Could you check a few things on this model? Use its own coordinates, in mm. Face numbers are marked on the shaded views. A direction names the side the tool comes from. Give positions to 0.01 mm unless a question says otherwise; leave off trailing zeros. Write each loop counter-clockwise with the first axis right and the second up, starting at its lowest first coordinate (ties: lowest second). Pieces come first, ordered by that corner, then holes. Notation, with made-up numbers: M 29.25,62 L 77.25,62 A32 cw 77.25,88 Z; hole C 12.25,6.5 d11. An arc over 180 degrees is marked long. Answer as a JSON object with one key per item and string values. Group by question number.
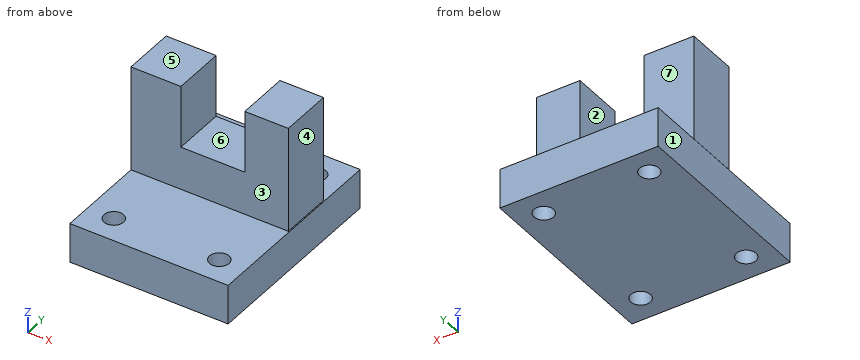
```python
from build123d import *

# Parameters (mm, degrees)
F2_W     = 0.0470026281
F2_H     = 25.4
F2_W_2   = 75.699427795
F3_DEPTH = 50.8
F1_W     = 76.2
F1_H     = 95.25
F1_R     = 4.699
F4_DEPTH = 19.05
F5_W     = 30.7534076273
F5_H     = 29.9894312948
F6_DEPTH = 31.75


with BuildPart() as f3:
    # F2 (on face) → F3 (new body)
    with BuildSketch(Plane.XY):
        with Locations((-24.0185575915, 19.0019719303)):
            Rectangle(F2_W, F2_H)
        with Locations((13.85465762, 19.0019719303)):
            Rectangle(F2_W_2, F2_H)
    extrude(amount=F3_DEPTH)

    # F1 (on face) → F4 (join)
    with BuildSketch(Plane.XY):
        with Locations((14.1049437225, 9.770923992)):
            Rectangle(F1_W, F1_H)
        with Locations((-11.2950562775, -25.154076008)):
            Circle(F1_R, mode=Mode.SUBTRACT)
        with Locations((39.5049437225, -25.154076008)):
            Circle(F1_R, mode=Mode.SUBTRACT)
        with Locations((-11.2950562775, 44.695923992)):
            Circle(F1_R, mode=Mode.SUBTRACT)
        with Locations((39.5049437225, 44.695923992)):
            Circle(F1_R, mode=Mode.SUBTRACT)
    extrude(amount=-F4_DEPTH)

    # F5 (on face) → F6 (cut)
    with BuildSketch(Plane.XZ.offset(-6.3019719303)):
        with Locations((15.3767038137, 35.8052843526)):
            Rectangle(F5_W, F5_H)
    extrude(amount=-F6_DEPTH, mode=Mode.SUBTRACT)


solid = f3.part
```
1) For the marked faces 5, 6 and 7, which set-ups out of +Z, -Z, +X, -X, +Y, -Y let a thin tool reach every point of the face, with its end or its side?
2) We'd pull the mould along X, two halves only. Please class the marked faces 1, 2, 3 and 4: released by +X, released by -X, zero draft, split by the parting line, or undercut.
3) If we section it at D-D, the plane y = 29: List the corners of the cut face in (x, z) for me.
4) If we section it at C-C, the plane x = -1.5: List the corners of the cut face in (y, z) for me.
5) Please list where these lines run through material, in increasing order: line 1 along X through (y, z) = (24.5, 36.5); line 2 along Y through (x, z) = (-15.5, 23); line 3 along Z through (x, y) = (12.5, 16). Write a range as from..to.
6) If we section it at B-B, the plane x = 42.5: List the corners of the cut face in (y, z) for me.
7) If we section it at A-A, the plane z = 28.5: List the corners of the cut face in (x, y) for me, plus the area to 3 significant figures.
8) I'm going to push flat-ended pins straight in: pin 1 (10 mm diameter, centred on x = 31.5, z = 32.5, fed in from +Y); pin 2 (7.5 mm diameter, centred on x = -11.3, y = 44.7, fed in from +Z); pin 3 (12.5 mm diameter, centred on y = 17.5, z = 20, fed in from +X); pin 4 (6 mm diameter, centred on x = 43, z = 12.5, fed in from -Y). Where does each tip first touch, or does it pass through?
Taken from the geometry:
{
 "1": {"face 5": "+Z, +X, -X, +Y, -Y", "face 6": "+Z, +Y, -Y", "face 7": "+Z, +X, -X, +Y"},
 "2": {"face 1": "released by -X", "face 2": "undercut", "face 3": "zero draft", "face 4": "released by +X"},
 "3": {"outline": "M -24.04,0 L -24,0 L -24,-19.05 L 52.2,-19.05 L 52.2,0 L 51.7,0 L 51.7,50.8 L 30.75,50.8 L 30.75,20.81 L 0,20.81 L 0,50.8 L -24.04,50.8 Z"},
 "4": {"outline": "M -37.85,-19.05 L 57.4,-19.05 L 57.4,0 L 31.7,0 L 31.7,50.8 L 6.3,50.8 L 6.3,0 L -37.85,0 Z"},
 "5": {"line 1": "-24.04..0, 30.75..51.7", "line 2": "6.3..31.7", "line 3": "-19.05..20.81"},
 "6": {"outline": "M -37.85,-19.05 L -28.77,-19.05 L -28.77,0 L -37.85,0 Z; M -21.53,-19.05 L 41.08,-19.05 L 41.08,0 L 31.7,0 L 31.7,50.8 L 6.3,50.8 L 6.3,0 L -21.53,0 Z; M 48.32,-19.05 L 57.4,-19.05 L 57.4,0 L 48.32,0 Z"},
 "7": {"outline": "M -24.04,6.3 L 0,6.3 L 0,31.7 L -24.04,31.7 Z; M 30.75,6.3 L 51.7,6.3 L 51.7,31.7 L 30.75,31.7 Z", "area": "1,140 mm²"},
 "8": {"pin 1": "y = 31.7", "pin 2": "through", "pin 3": "x = 51.7", "pin 4": "y = 6.3"}
}
